Work out the finished part from the listing and answer in its coordinate system (mm). Face numbers are marked on the shaded views. A direction names the side the tool comes from. Give positions to 0.01 mm unless a question says otherwise; leave off trailing zeros. Order: outer loops, then holes, each group sorted by start corner. A loop starts at its lowest first (then second) coordinate and runs counter-clockwise, first axis right, second up. Notation, with made-up numbers: (-27, -14.5) - (17, -14.5) arc R30 ccw to (17, 21.5) - close; hole circle Ø1 at (-19, 85.25). An arc over 180 degrees is marked (long way). Put each result on its own line as item: value.
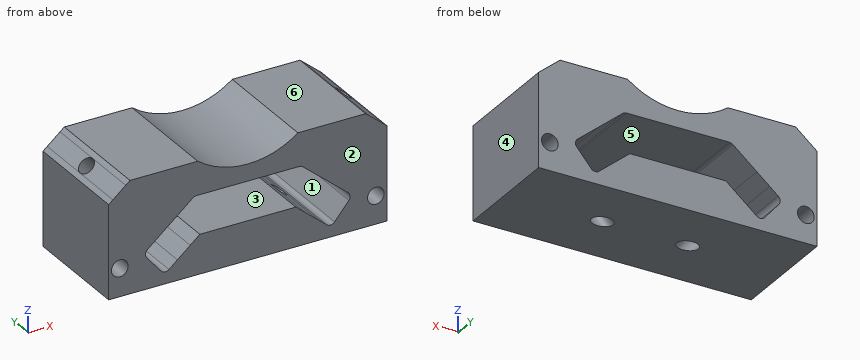
```python
from build123d import *

# Parameters (mm, degrees)
F0_R     = 1.5
F1_DEPTH = 10
F2_R     = 1.5
F3_DEPTH = 44.9992499642
F4_R     = 1.5
F5_DEPTH = 44.9992499642


with BuildPart() as f1:
    # F0 (on Front) → F1 (new body, symmetric)
    with BuildSketch(Plane.XZ):
        with BuildLine():
            Line((9.6094143182, -10), (25, -10))
            Line((25, -10), (25, 6.7860619516))
            Line((25, 6.7860619516), (24.2339555569, 7.4288495613))
            Line((24.2339555569, 7.4288495613), (16.5025435388, -1.7850884872))
            Line((16.5025435388, -1.7850884872), (18.034632425, -3.0706637066))
            ThreePointArc((18.034632425, -3.0706637066), (18.3880395134, -3.7495524069), (18.1578892584, -4.4794957594))
            Line((18.1578892584, -4.4794957594), (15.5867388197, -7.5436735318))
            ThreePointArc((15.5867388197, -7.5436735318), (14.9078501193, -7.8970806202), (14.1779067669, -7.6669303653))
            Line((14.1779067669, -7.6669303653), (12.6458178806, -6.3813551459))
            Line((12.6458178806, -6.3813551459), (9.6094143182, -10))
        make_face()
        with Locations((23, -5)):
            Circle(F0_R, mode=Mode.SUBTRACT)
        Polygon((5.6931924502, -10), (9.6094143182, -10), (12.6458178806, -6.3813551459), (10.3476845513, -4.4529923168), align=None)
        Polygon((-5.6931924502, -10), (5.6931924502, -10), (10.3476845513, -4.4529923168), (8.6160757377, -3), (0, -3), (-8.6160757377, -3), (-10.3476845513, -4.4529923168), align=None)
        Polygon((16.5025435388, -1.7850884872), (24.2339555569, 7.4288495613), (21.9358222275, 9.3572123903), (14.2044102094, 0.1432743419), align=None)
        Polygon((-9.6094143182, -10), (-5.6931924502, -10), (-10.3476845513, -4.4529923168), (-12.6458178806, -6.3813551459), align=None)
        with BuildLine():
            Line((14.2044102094, 0.1432743419), (21.9358222275, 9.3572123903))
            Line((21.9358222275, 9.3572123903), (21.1697777844, 10))
            Line((21.1697777844, 10), (9, 10))
            ThreePointArc((9, 10), (4.7434164903, 7.7697505292), (0, 7))
            ThreePointArc((0, 7), (-4.7434164903, 7.7697505292), (-9, 10))
            Line((-9, 10), (-21.1697777844, 10))
            Line((-21.1697777844, 10), (-21.9358222275, 9.3572123903))
            Line((-21.9358222275, 9.3572123903), (-14.2044102094, 0.1432743419))
            Line((-14.2044102094, 0.1432743419), (-9.8869609261, 3.7660444431))
            ThreePointArc((-9.8869609261, 3.7660444431), (-9.5861934597, 3.9396926208), (-9.2441733164, 4))
            Line((-9.2441733164, 4), (0, 4))
            Line((0, 4), (9.2441733164, 4))
            ThreePointArc((9.2441733164, 4), (9.5861934597, 3.9396926208), (9.8869609261, 3.7660444431))
            Line((9.8869609261, 3.7660444431), (14.2044102094, 0.1432743419))
        make_face()
        with BuildLine():
            Line((-25, -10), (-9.6094143182, -10))
            Line((-9.6094143182, -10), (-12.6458178806, -6.3813551459))
            Line((-12.6458178806, -6.3813551459), (-14.1779067669, -7.6669303653))
            ThreePointArc((-14.1779067669, -7.6669303653), (-14.9078501193, -7.8970806202), (-15.5867388197, -7.5436735318))
            Line((-15.5867388197, -7.5436735318), (-18.1578892584, -4.4794957594))
            ThreePointArc((-18.1578892584, -4.4794957594), (-18.3880395134, -3.7495524069), (-18.034632425, -3.0706637066))
            Line((-18.034632425, -3.0706637066), (-16.5025435388, -1.7850884872))
            Line((-16.5025435388, -1.7850884872), (-24.2339555569, 7.4288495613))
            Line((-24.2339555569, 7.4288495613), (-25, 6.7860619516))
            Line((-25, 6.7860619516), (-25, -10))
        make_face()
        with Locations((-23, -5)):
            Circle(F0_R, mode=Mode.SUBTRACT)
        Polygon((-16.5025435388, -1.7850884872), (-14.2044102094, 0.1432743419), (-21.9358222275, 9.3572123903), (-24.2339555569, 7.4288495613), align=None)
    extrude(amount=F1_DEPTH, both=True)

    # F2 (on face) → F3 (cut, through all)
    with BuildSketch(Plane(origin=(-13.6708809903, 0, 16.2923215341), x_dir=(0.7660444431, 0, 0.6427876097), z_dir=(-0.6427876097, 0, 0.7660444431))):
        with Locations((-12.2891145369, 0)):
            Circle(F2_R)
    extrude(amount=-F3_DEPTH, mode=Mode.SUBTRACT)

    # F4 (on face) → F5 (cut, through all)
    with BuildSketch(Plane(origin=(13.6708809903, 0, 16.2923215341), x_dir=(0.7660444431, 0, -0.6427876097), z_dir=(0.6427876097, 0, 0.7660444431))):
        with Locations((12.2891145369, 0)):
            Circle(F4_R)
    extrude(amount=-F5_DEPTH, mode=Mode.SUBTRACT)


solid = f1.part
```
(1) A tool of negligible diameter and unlimited length cuts with its end or side. For the marked faces 1 and 2, from which of +Z, -Z, +X, -X, +Y, -Y can it reach the whole face along a straight path? Write none if from no direction.
Geometry check:
face 1: +Y, -Y
face 2: +Z, -Z, +X, -X, -Y
(2) Determine the mould class of the marked faces 3, 4, 5 and 6 for opening direction X: pulls with the +X half, pulls with the -X half, needs draft (parallel to the pull), parting line crosses it, or undercut.
Geometry check:
face 3: undercut
face 4: pulls with the +X half
face 5: undercut
face 6: needs draft
(3) Section A-A, the plane x = 17 is taken. Count the separate pieces of the cut face and the enclosed holes in it, then the cut area to 3 significant figures.
Geometry check:
separate pieces: 2
enclosed holes: 1
area: 316 mm²
(4) Straight lines are drawn through the part: line 1 (X direction, y = -6.25, z = -7.5); line 2 (Z direction, x = -15, y = 8); line 3 (Z direction, x = 23, y = 4.5). For each, find the intervals that lie inside material, in ascending order.
Geometry check:
line 1: x = -25 to -15.62, -13.98 to 13.98, 15.62 to 25
line 2: z = -10 to -7.88, -0.52 to 10
line 3: z = -10 to -6.5, -3.5 to 8.46
(5) Section C-C, the plane y = 4.25 is taken. Write down the section's boundary in (x, z), then the cut area to 3 significant figures.
Geometry check:
outline: (-25, -10) - (25, -10) - (25, 6.79) - (21.17, 10) - (9, 10) arc R15 cw to (-9, 10) - (-21.17, 10) - (-25, 6.79) - close; hole circle Ø3 at (-23, -5); hole (-18.16, -4.48) - (-15.59, -7.54) arc R1 ccw to (-14.18, -7.67) - (-8.62, -3) - (8.62, -3) - (14.18, -7.67) arc R1 ccw to (15.59, -7.54) - (18.16, -4.48) arc R1 ccw to (18.03, -3.07) - (9.89, 3.77) arc R1 ccw to (9.24, 4) - (-9.24, 4) arc R1 ccw to (-9.89, 3.77) - (-18.03, -3.07) arc R1 ccw to start; hole circle Ø3 at (23, -5)
area: 689 mm²
(6) Given pin 1 (2.5 mm diameter, centred on x = -23, z = -5, fed in from -Y); pin 2 (4 mm diameter, centred on x = 23, z = -5, fed in from +Y); pin 3 (5 mm diameter, centred on x = 2.5, y = -2, fed in from +Z), each flat-ended and moving along its own axis, determine where each tip first touches the part or whether it passes through.
Geometry check:
pin 1: passes through
pin 2: stops at y = 10
pin 3: stops at z = 7.86
